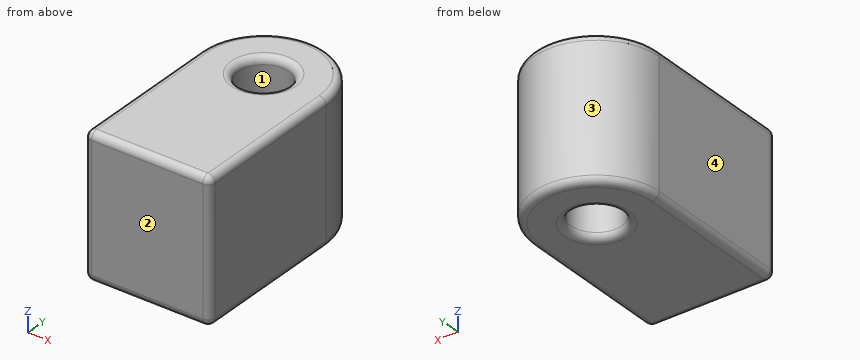
```python
from build123d import *

# Parameters (mm, degrees)
F0_R     = 17.948255
F1_DEPTH = 100
F2_R     = 5
F3_R     = 5


with BuildPart() as f1:
    # F0 (on Top) → F1 (new body)
    with BuildSketch(Plane.XY):
        with BuildLine():
            ThreePointArc((36.747999, 35.844807), (-7.825233, 80.418039), (-52.398466, 35.844807))
            Line((-52.398466, 35.844807), (-52.398466, -74.351192))
            Line((-52.398466, -74.351192), (36.747999, -74.351192))
            Line((36.747999, -74.351192), (36.747999, 35.844807))
        make_face()
        with Locations((-7.825233, 35.844807)):
            Circle(F0_R, mode=Mode.SUBTRACT)
    extrude(amount=F1_DEPTH)

    # F2
    f2_edges = [f1.edges().sort_by_distance(p)[0] for p in [
        (-7.825233, 80.418039, 0),
        (36.747999, -19.253192, 100),
        (-7.825233, 80.418039, 100),
        (36.747999, -74.351192, 50),
        (-52.398466, -19.253192, 100),
        (-52.398466, -19.253192, 0),
        (-7.825233, -74.351192, 0),
        (-52.398466, -74.351192, 50),
        (-7.825233, -74.351192, 100),
        (36.747999, -19.253192, 0),
    ]]
    fillet(f2_edges, radius=F2_R)

    # F3
    f3_edges = [f1.edges().sort_by_distance(p)[0] for p in [
        (-25.773488, 35.844807, 100),
        (-25.773488, 35.844807, 0),
    ]]
    fillet(f3_edges, radius=F3_R)


solid = f1.part
```
Could you check a few things on this model? Use its own coordinates, in mm. Face numbers are marked on the shaded views. Coordinates: 2 decimals unless noted, no trailing zeros. Write each loop counter-clockwise with the first axis right and the second up, starting at its lowest first coordinate (ties: lowest second). Pieces come first, ordered by that corner, then holes. Notation, with made-up numbers: M 39.25,56.25 L 64.25,56.25 A20 cw 64.25,73.25 Z; hole C -12.75,70.5 d6. An arc over 180 degrees is marked long. Answer as CSV lines item,"result". Start each with the question number.
1) I want a section at A-A, the plane z = 48. Please give me the cut outline in (x, y), and give its area (3 significant figures).
2) For P1, Ø2, axis at x = -28.5, y = 38.5, coming from the +Z side; P2, Ø4, axis at x = 26, y = 61, coming from the -Z side; P3, Ø1, axis at x = -4, z = 75.5, coming from the +Y side, each with a flat end and sliding along its axis, tell me the tip position at first contact or that it passes through.
3) We'd pull the mould along X, two halves only. Please class the marked faces 1, 2, 3 and 4: +X half, -X half, draft (parallel to the pull), parting line (faces both ways), or undercut.
4) Please list where these lines run through material, in increasing order: line 1 (Y direction, x = -19.5, z = 25.5); line 2 (X direction, y = 45, z = 9); line 3 (Y direction, x = -3, z = 39). Write a range as from..to.
Data:
1,outline,"M -52.4,-69.35 A5 ccw -47.4,-74.35 L 31.75,-74.35 A5 ccw 36.75,-69.35 L 36.75,35.84 A44.57 ccw -52.4,35.84 Z; hole C -7.83,35.84 d35.9"
1,area,"11,900 mm^2"
2,P1,"stops at z = 99.88"
2,P2,"stops at z = 0.03"
2,P3,"stops at y = 80.29"
3,face 1,"undercut"
3,face 2,"draft"
3,face 3,"parting line"
3,face 4,"-X half"
4,line 1,"y = -74.35..22.21, 49.48..78.86"
4,line 2,"x = -51.45..-23.26, 7.61..35.8"
4,line 3,"y = -74.35..18.56, 53.13..80.16"
